from build123d import *

# Parameters (mm, degrees)
SKETCH5_R           = 13
BOSS_EXTRUDE3_DEPTH = 3
SKETCH6_W           = 6.5
SKETCH6_H           = 20
BOSS_EXTRUDE4_DEPTH = 3
BOSS_EXTRUDE5_DEPTH = 3
SKETCH9_R           = 1.75
CUT_EXTRUDE1_DEPTH  = 3
FILLET1_R           = 2


with BuildPart() as part:
    # Sketch5 → Boss-Extrude3 (new body)
    with BuildSketch(Plane.XY.offset(3)):
        with Locations((0, 20.92523633)):
            Circle(SKETCH5_R)
    extrude(amount=BOSS_EXTRUDE3_DEPTH)

    # Sketch6 → Boss-Extrude4 (add)
    with BuildSketch(Plane.XY.offset(3)):
        with Locations((0.239986303, 43.081718219)):
            Rectangle(SKETCH6_W, SKETCH6_H)
    extrude(amount=BOSS_EXTRUDE4_DEPTH)

    # Sketch8 → Boss-Extrude5 (add)
    with BuildSketch(Plane.XY.offset(3)):
        with BuildLine():
            Line((-4.295994306, 33.146239501), (-3.38996239, 33.41049881))
            ThreePointArc((-3.38996239, 33.41049881), (-3.583611793, 34.300219718), (-4.075784869, 35.066293507))
            ThreePointArc((-4.075784869, 35.066293507), (-4.733344139, 35.009325085), (-4.939904397, 34.382457909))
            ThreePointArc((-4.939904397, 34.382457909), (-4.746199027, 33.697547192), (-4.295994306, 33.146239501))
        make_face()
        with BuildLine():
            Line((-6.479661136, 32.095481488), (-5.638197922, 32.522876474))
            ThreePointArc((-5.638197922, 32.522876474), (-5.993184011, 33.36138006), (-6.618649024, 34.023117852))
            ThreePointArc((-6.618649024, 34.023117852), (-7.254301529, 33.845422924), (-7.341262628, 33.191154353))
            ThreePointArc((-7.341262628, 33.191154353), (-7.024130865, 32.55393233), (-6.479661136, 32.095481488))
        make_face()
        with BuildLine():
            Line((-8.431105641, 30.65869425), (-7.68329101, 31.234454696))
            ThreePointArc((-7.68329101, 31.234454696), (-8.187345926, 31.992763359), (-8.924487613, 32.527296351))
            ThreePointArc((-8.924487613, 32.527296351), (-9.516266026, 32.235015826), (-9.480622702, 31.575956535))
            ThreePointArc((-9.480622702, 31.575956535), (-9.05102421, 31.008444775), (-8.431105641, 30.65869425))
        make_face()
        with BuildLine():
            Line((-10.082888425, 28.885531296), (-9.454565882, 29.589759666))
            ThreePointArc((-9.454565882, 29.589759666), (-10.090270139, 30.241667239), (-10.913613837, 30.630522663))
            ThreePointArc((-10.913613837, 30.630522663), (-11.44106706, 30.233757376), (-11.284051101, 29.592683602))
            ThreePointArc((-11.284051101, 29.592683602), (-10.756832248, 29.114494578), (-10.082888425, 28.885531296))
        make_face()
        with BuildLine():
            Line((-11.377926009, 26.837270843), (-10.89080957, 27.645629915))
            ThreePointArc((-10.89080957, 27.645629915), (-11.63619405, 28.168607317), (-12.517286067, 28.398346832))
            ThreePointArc((-12.517286067, 28.398346832), (-12.962185999, 27.910808479), (-12.689223673, 27.309874902))
            ThreePointArc((-12.689223673, 27.309874902), (-12.08260446, 26.937534209), (-11.377926009, 26.837270843))
        make_face()
        with BuildLine():
            Line((-12.271463571, 24.584698125), (-11.942387349, 25.469252055))
            ThreePointArc((-11.942387349, 25.469252055), (-12.77169253, 25.845225862), (-13.680083464, 25.907909968))
            ThreePointArc((-13.680083464, 25.907909968), (-14.027054939, 25.346447244), (-13.647579472, 24.806421351))
            ThreePointArc((-13.647579472, 24.806421351), (-12.982523874, 24.5527966), (-12.271463571, 24.584698125))
        make_face()
        with BuildLine():
            Line((-12.732621608, 22.20565914), (-12.572958051, 23.135838888))
            ThreePointArc((-12.572958051, 23.135838888), (-13.457524218, 23.351815933), (-14.361821254, 23.245278348))
            ThreePointArc((-14.361821254, 23.245278348), (-14.598873387, 22.629294678), (-14.125998959, 22.168839065))
            ThreePointArc((-14.125998959, 22.168839065), (-13.425490439, 22.042695201), (-12.732621608, 22.20565914))
        make_face()
        with BuildLine():
            Line((-12.745463094, 19.782370399), (-12.76072997, 20.726030156))
            ThreePointArc((-12.76072997, 20.726030156), (-13.669987659, 20.774546551), (-14.538939462, 20.502469076))
            ThreePointArc((-14.538939462, 20.502469076), (-14.657880036, 19.853252059), (-14.107948577, 19.488279478))
            ThreePointArc((-14.107948577, 19.488279478), (-13.396195802, 19.493975869), (-12.745463094, 19.782370399))
        make_face()
        with BuildLine():
            Line((-12.309544245, 17.398577627), (-12.499213949, 18.323105732))
            ThreePointArc((-12.499213949, 18.323105732), (-13.401740392, 18.202484813), (-14.20531711, 17.774270094))
            ThreePointArc((-14.20531711, 17.774270094), (-14.202035694, 17.114255831), (-13.594052123, 16.857379261))
            ThreePointArc((-13.594052123, 16.857379261), (-12.895652349, 16.994719047), (-12.309544245, 17.398577627))
        make_face()
        with BuildLine():
            Line((-11.439929852, 15.136661617), (-11.797447644, 16.010107576))
            ThreePointArc((-11.797447644, 16.010107576), (-12.662052694, 15.724517845), (-13.372483756, 15.154964429))
            ThreePointArc((-13.372483756, 15.154964429), (-13.247093752, 14.506962159), (-12.602069194, 14.367058922))
            ThreePointArc((-12.602069194, 14.367058922), (-11.941158214, 14.631295818), (-11.439929852, 15.136661617))
        make_face()
        with BuildLine():
            Line((-10.166672663, 13.074791263), (-10.679683192, 13.866969912))
            ThreePointArc((-10.679683192, 13.866969912), (-11.476487216, 13.426280982), (-12.069221043, 12.735071898))
            ThreePointArc((-12.069221043, 12.735071898), (-11.826055767, 12.121475741), (-11.166281438, 12.103380713))
            ThreePointArc((-11.166281438, 12.103380713), (-10.565699479, 12.485383033), (-10.166672663, 13.074791263))
        make_face()
        with BuildLine():
            Line((-8.533774801, 11.284222136), (-9.184549085, 11.967756807))
            ThreePointArc((-9.184549085, 11.967756807), (-9.886015568, 11.387198317), (-10.340568045, 10.598220857))
            ThreePointArc((-10.340568045, 10.598220857), (-9.988030974, 10.040235902), (-9.336307821, 10.144574423))
            ThreePointArc((-9.336307821, 10.144574423), (-8.816810221, 10.631140662), (-8.533774801, 11.284222136))
        make_face()
        with BuildLine():
            Line((-6.597667103, 9.826833991), (-7.363715226, 10.378102608))
            ThreePointArc((-7.363715226, 10.378102608), (-7.945602392, 9.677737908), (-8.246264774, 8.818258113))
            ThreePointArc((-8.246264774, 8.818258113), (-7.796539134, 8.3351676), (-7.175389866, 8.558333865))
            ThreePointArc((-7.175389866, 8.558333865), (-6.754929788, 9.132648922), (-6.597667103, 9.826833991))
        make_face()
        with BuildLine():
            Line((-4.425258947, 8.752992275), (-5.280107276, 9.152943708))
            ThreePointArc((-5.280107276, 9.152943708), (-5.722305859, 8.356976498), (-5.858687642, 7.456696877))
            ThreePointArc((-5.858687642, 7.456696877), (-5.327315369, 7.065195788), (-4.758206101, 7.399477461))
            ThreePointArc((-4.758206101, 7.399477461), (-4.451314103, 8.041693751), (-4.425258947, 8.752992275))
        make_face()
        with BuildLine():
            Line((-2.091625949, 8.09980757), (-3.005732032, 8.334620015))
            ThreePointArc((-3.005732032, 8.334620015), (-3.292960219, 7.470557891), (-3.260348227, 6.560590944))
            ThreePointArc((-3.260348227, 6.560590944), (-2.665692859, 6.274209051), (-2.168291272, 6.708053788))
            ThreePointArc((-2.168291272, 6.708053788), (-1.985573144, 7.395977147), (-2.091625949, 8.09980757))
        make_face()
        with BuildLine():
            Line((0.322584552, 7.889853094), (-0.61918896, 7.951411738))
            ThreePointArc((-0.61918896, 7.951411738), (-0.741520518, 7.049115568), (-0.541041777, 6.160908576))
            ThreePointArc((-0.541041777, 6.160908576), (0.096346165, 5.989542866), (0.504850516, 6.507957556))
            ThreePointArc((0.504850516, 6.507957556), (0.557080271, 7.217814242), (0.322584552, 7.889853094))
        make_face()
    extrude(amount=BOSS_EXTRUDE5_DEPTH)

    # Sketch9 → Cut-Extrude1 (cut)
    with BuildSketch(Plane(origin=(0, 0, 3), x_dir=(-1, 0, 0), z_dir=(0, 0, -1))):
        with Locations((-0.239986303, 49.531718219)):
            Circle(SKETCH9_R)
        with Locations((-0.239986303, 20.92523633)):
            Circle(SKETCH9_R)
    extrude(amount=-CUT_EXTRUDE1_DEPTH, mode=Mode.SUBTRACT)

    # Fillet1
    fillet1_edges = [part.edges().sort_by_distance(p)[0] for p in [
        (-3.010013697, 53.081718219, 4.5),
        (3.489986303, 53.081718219, 4.5),
    ]]
    fillet(fillet1_edges, radius=FILLET1_R)


solid = part.part
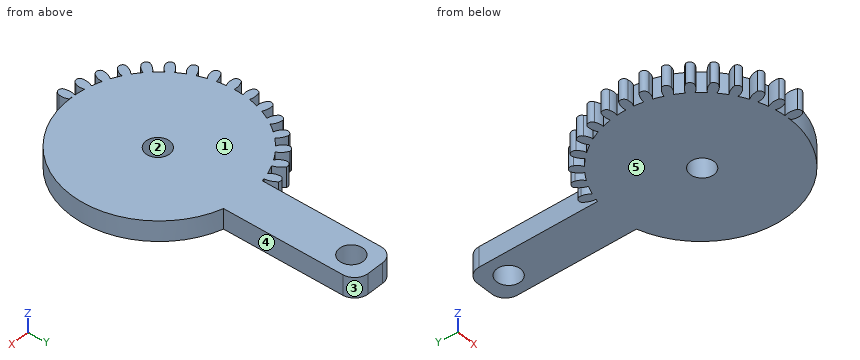
Source: CAD feature listing. Evaluate the final solid. Frame: model axes, mm. Face numbers are marked on the shaded views. A direction names the side the tool comes from. Round coordinates to 2 decimals unless told otherwise and drop trailing zeros. Loops run counter-clockwise (first coordinate to the right, second up) from the corner with the lowest first, then second, coordinate; pieces in that order, holes last.
Q1. Section D-D, the plane x = 10.25. Return loops of the section in (y, z), plus the area to 3 significant figures.
Q2. Section B-B, the plane y = 42.5. Return loops of the section in (x, z).
Q3. Section C-C, the plane z = 3.55. State how many separate pieces and enclosed holes the cut face has, plus the area to 3 significant figures.
Q4. Access query for the marked faces 4 and 5. Directions: +Z, -Z, +X, -X, +Y, -Y. A direction counts if a zero-diameter tool reaches every point of the face in a straight line with its end or side. Return the directions, or none.
Q5. Mould query, pull axis Y, two halves, no side actions, for the marked faces 1, 2 and 3. Classes: pulls with the +Y half, pulls with the -Y half, needs draft (parallel to the pull), parting line crosses it, or undercut.
Q6. Ray query, line 1 (Y direction, x = 1.25, z = 3.15); line 2 (Y direction, x = 0.75, z = 3.65); line 3 (X direction, y = 31.5, z = 4.4). Return the intervals inside material, ascending.
Q7. First-contact query: P1, Ø0.9, axis at y = 45.5, z = 5, coming from the -X side. Flat tip, straight axial feed; report the tip coordinate or a pass-through.
Q8. Section A-A, the plane y = 49. Return loops of the section in (x, z), plus the area to 3 significant figures.
Solutions:
1. outline: (12.93, 3) - (28.92, 3) - (28.92, 6) - (12.93, 6) - close
1. area: 48.0 mm2
2. outline: (-3.01, 3) - (3.49, 3) - (3.49, 6) - (-3.01, 6) - close
3. separate pieces: 1
3. enclosed holes: 2
3. area: 668 mm2
4. face 4: +Z, -Z, +X, +Y
4. face 5: -Z, +X, -X, +Y, -Y
5. face 1: needs draft
5. face 2: undercut
5. face 3: pulls with the +Y half
6. line 1: y = 7.99 to 19.5, 22.35 to 48.1, 50.96 to 53.08
6. line 2: y = 7.95 to 19.25, 22.6 to 47.86, 51.21 to 53.08
6. line 3: x = -9.44 to -7.82, -7.56 to 7.56
7. P1: stops at x = -3.01
8. outline: (-3.01, 3) - (-1.43, 3) - (-1.43, 6) - (-3.01, 6) - close; (1.91, 3) - (3.49, 3) - (3.49, 6) - (1.91, 6) - close
8. area: 9.50 mm2
